from build123d import *

# Parameters (mm, degrees)
F0_W           = 76.2
F0_H           = 35.56
F1_DEPTH       = 71.12
F0_H_2         = 76.2
F2_DEPTH       = 35.56
F4_DEPTH       = 76.2
F6_D           = 15.24
F6_CBORE_D     = 40.64
F6_CBORE_DEPTH = 10.16
F8_DEPTH       = 27.94
F10_DEPTH      = 10.16
F11_R          = 10.16


with BuildPart() as f1:
    # F0 (on Top) → F1 (new body)
    with BuildSketch(Plane.XY):
        with Locations((38.1, 129.54)):
            Rectangle(F0_W, F0_H)
        with Locations((38.1, 93.98)):
            Rectangle(F0_W, F0_H)
    extrude(amount=F1_DEPTH)

    # F0 (on Top) → F2 (join)
    with BuildSketch(Plane.XY):
        with Locations((38.1, 38.1)):
            Rectangle(F0_W, F0_H_2)
    extrude(amount=F2_DEPTH)

    # F3 (on face) → F4 (cut)
    with BuildSketch(Plane.YZ.offset(76.2)):
        Polygon((76.2, 71.12), (76.2, 35.56), (111.76, 71.12), align=None)
        Polygon((147.32, 0), (147.32, 35.56), (111.76, 0), align=None)
    extrude(amount=-F4_DEPTH, mode=Mode.SUBTRACT)

    # F6 (through all)
    with Locations(Plane.XY.offset(35.56)):
        with Locations((38.1, 38.1)):
            CounterBoreHole(F6_D / 2, F6_CBORE_D / 2, F6_CBORE_DEPTH)

    # F7 (on face) → F8 (cut)
    with BuildSketch(Plane.XY.offset(71.12)):
        with BuildLine():
            Line((60.96, 137.16), (15.24, 137.16))
            ThreePointArc((15.24, 137.16), (7.62, 129.54), (15.24, 121.92))
            Line((15.24, 121.92), (60.96, 121.92))
            ThreePointArc((60.96, 121.92), (68.58, 129.54), (60.96, 137.16))
        make_face()
    extrude(amount=-F8_DEPTH, mode=Mode.SUBTRACT)

    # F9 (on face) → F10 (cut)
    with BuildSketch(Plane.XY.offset(35.56)):
        with BuildLine():
            Line((43.18, 76.2), (33.02, 76.2))
            Line((33.02, 76.2), (33.02, 57.7747553987))
            ThreePointArc((33.02, 57.7747553987), (38.1, 58.42), (43.18, 57.7747553987))
            Line((43.18, 57.7747553987), (43.18, 76.2))
        make_face()
        with BuildLine():
            ThreePointArc((43.18, 18.4252446013), (38.1, 17.78), (33.02, 18.4252446013))
            Line((33.02, 18.4252446013), (33.02, 0))
            Line((33.02, 0), (43.18, 0))
            Line((43.18, 0), (43.18, 18.4252446013))
        make_face()
    extrude(amount=-F10_DEPTH, mode=Mode.SUBTRACT)

    # F11
    f11_edges = [f1.edges().sort_by_distance(p)[0] for p in [
        (76.2, 0, 17.78),
        (0, 0, 17.78),
    ]]
    fillet(f11_edges, radius=F11_R)


solid = f1.part
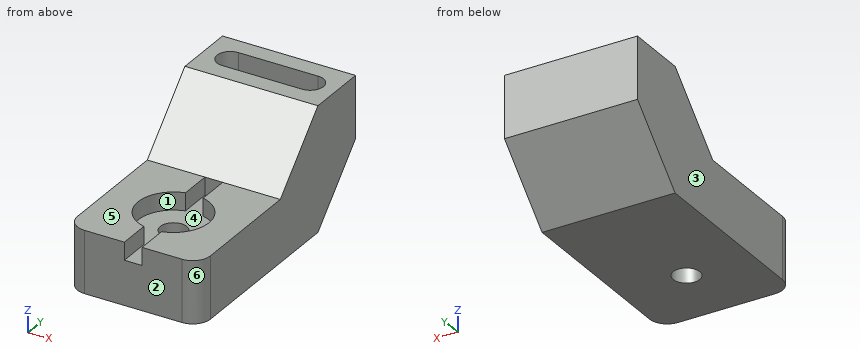
The model under review builds one solid part; all positions refer to its coordinate system, in mm. Face numbers are marked on the shaded views. A direction names the side the tool comes from. Give positions to 0.01 mm unless a question says otherwise; leave off trailing zeros. Order: outer loops, then holes, each group sorted by start corner. A loop starts at its lowest first (then second) coordinate and runs counter-clockwise, first axis right, second up. Notation, with made-up numbers: M -0.75,-26.75 L 32.25,-26.75 A7 cw 32.25,-22.75 Z; hole C 63,61 d2. An arc over 180 degrees is marked long. Use one line per item in the form item = value. Start each with the question number.
Item 1: We need section B-B on x = 38.1. Give the boundary of the cut face in (y, z), plus the area to 3 significant figures.
Item 2: For the marked faces 4, 5 and 6, list the 3-axis set-ups (+Z, -Z, +X, -X, +Y, -Y) from which the entire face can be reached by the end or side of a thin tool; tool diameter is ignored.
Item 3: We need section C-C on z = 67.5. Give the boundary of the cut face in (x, y).
Item 4: The part is to be moulded in two halves that separate along Y. For the marked faces 1, 2 and 3, say which applies: pulls with the +Y half, pulls with the -Y half, needs draft (parallel to the pull), parting line crosses it, or undercut.
Item 5: Insertion check: pin 1 Ø9 at (x, y) = (38.1, 38.1) entering from -Z; pin 2 Ø11 at (y, z) = (9, 32) entering from +X; pin 3 Ø20.5 at (x, y) = (44.5, 40.5) entering from +Z; pin 4 Ø10 at (x, y) = (66.5, 54.5) entering from +Z. Each pin has a flat end and moves straight along its axis. Give the tip position at first contact, or say it passes through.
Item 6: To check wall thickness, follow line 1 along X through (y, z) = (38, 14); line 2 along Z through (x, y) = (58, 76); line 3 along Z through (x, y) = (31.5, 48.5). State the ranges of each line that lie inside material, in increasing order. Write a range as from..to.
Item 7: We need section D-D on y = 71. Give the boundary of the cut face in (x, z).
Item 8: We need section A-A on y = 38.1. Give the boundary of the cut face in (x, z).
Completed:
q1.outline = M 0,0 L 30.48,0 L 30.48,25.4 L 0,25.4 Z; M 45.72,0 L 111.76,0 L 147.32,35.56 L 147.32,71.12 L 137.16,71.12 L 137.16,43.18 L 121.92,43.18 L 121.92,71.12 L 111.76,71.12 L 76.2,35.56 L 76.2,25.4 L 45.72,25.4 Z
q1.area = 4,920 mm²
q2.face_4 = +Z
q2.face_5 = +Z, +X, -X, -Y
q2.face_6 = +Z, -Z, +X, -Y
q3.outline = M 0,108.14 L 76.2,108.14 L 76.2,147.32 L 0,147.32 Z; hole M 15.24,121.92 L 60.96,121.92 A7.62 ccw 60.96,137.16 L 15.24,137.16 A7.62 ccw Z
q4.face_1 = undercut
q4.face_2 = pulls with the -Y half
q4.face_3 = needs draft
q5.pin_1 = through
q5.pin_2 = 76.2
q5.pin_3 = 25.4
q5.pin_4 = 35.56
q6.line_1 = 0..30.48, 45.72..76.2
q6.line_2 = 0..35.56
q6.line_3 = 0..25.4
q7.outline = M 0,0 L 76.2,0 L 76.2,35.56 L 43.18,35.56 L 43.18,25.4 L 33.02,25.4 L 33.02,35.56 L 0,35.56 Z
q8.outline = M 0,0 L 30.48,0 L 30.48,25.4 L 17.78,25.4 L 17.78,35.56 L 0,35.56 Z; M 45.72,0 L 76.2,0 L 76.2,35.56 L 58.42,35.56 L 58.42,25.4 L 45.72,25.4 Z
